Part model, mm, in its own coordinate system. Face numbers are marked on the shaded views. A direction names the side the tool comes from. Give positions to 0.01 mm unless a question says otherwise; leave off trailing zeros. Loops run counter-clockwise (first coordinate to the right, second up) from the corner with the lowest first, then second, coordinate; pieces in that order, holes last. Notation, with made-up numbers: M -38,-16 L 10,-16 A15 ccw 10,1 Z; hole C -17.75,85.25 d3. An arc over 180 degrees is marked long. Answer in a Markdown table with one row per item.
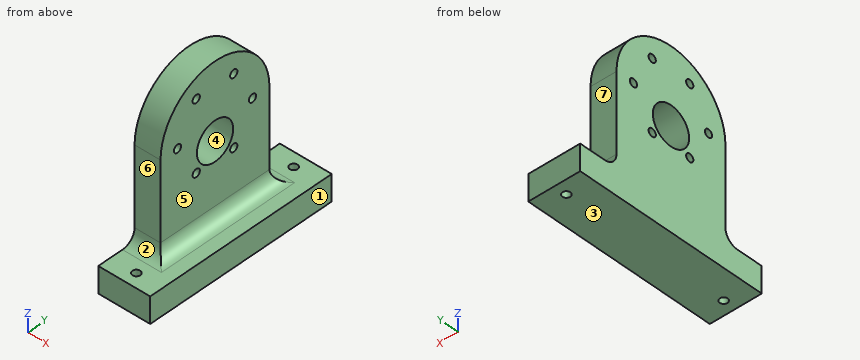
from build123d import *

# Parameters (mm, degrees)
SKETCH1_R           = 7.5
SKETCH1_R_2         = 1.5
BOSS_EXTRUDE1_DEPTH = 10
FILLET1_R           = 5
FILLET2_R           = 5
SKETCH2_W           = 10
SKETCH2_H           = 75
BOSS_EXTRUDE2_DEPTH = 10
FILLET3_R           = 5
SKETCH3_R           = 1.5
CUT_EXTRUDE1_DEPTH  = 10


with BuildPart() as part:
    # Sketch1 → Boss-Extrude1 (new body)
    with BuildSketch(Plane(origin=(0, 0, 0), x_dir=(0, 0, -1), z_dir=(1, 0, 0))):
        with BuildLine():
            Line((0, 0), (35, 0))
            Line((35, 0), (35, -15))
            Line((35, -15), (45, -15))
            Line((45, -15), (45, 60))
            Line((45, 60), (35, 60))
            Line((35, 60), (35, 45))
            Line((35, 45), (0, 45))
            ThreePointArc((0, 45), (-22.5, 22.5), (0, 0))
        make_face()
        with Locations((6.423393759, 22.5)):
            Circle(SKETCH1_R, mode=Mode.SUBTRACT)
        with Locations((13.423393759, 30.25)):
            Circle(SKETCH1_R_2, mode=Mode.SUBTRACT)
        with Locations((0, 38)):
            Circle(SKETCH1_R_2, mode=Mode.SUBTRACT)
        with Locations((-13.423393759, 30.25)):
            Circle(SKETCH1_R_2, mode=Mode.SUBTRACT)
        with Locations((-13.423393759, 14.75)):
            Circle(SKETCH1_R_2, mode=Mode.SUBTRACT)
        with Locations((0, 7)):
            Circle(SKETCH1_R_2, mode=Mode.SUBTRACT)
        with Locations((13.423393759, 14.75)):
            Circle(SKETCH1_R_2, mode=Mode.SUBTRACT)
    extrude(amount=BOSS_EXTRUDE1_DEPTH)

    # Fillet1
    fillet1_edges = [part.edges().sort_by_distance(p)[0] for p in [
        (5, 45, -35),
    ]]
    fillet(fillet1_edges, radius=FILLET1_R)

    # Fillet2
    fillet2_edges = [part.edges().sort_by_distance(p)[0] for p in [
        (5, 0, -35),
    ]]
    fillet(fillet2_edges, radius=FILLET2_R)

    # Sketch2 → Boss-Extrude2 (add)
    with BuildSketch(Plane(origin=(10, 0, 0), x_dir=(0, 0, -1), z_dir=(1, 0, 0))):
        with Locations((40, 22.5)):
            Rectangle(SKETCH2_W, SKETCH2_H)
    extrude(amount=BOSS_EXTRUDE2_DEPTH)

    # Fillet3
    fillet3_edges = [part.edges().sort_by_distance(p)[0] for p in [
        (10, 22.5, -35),
    ]]
    fillet(fillet3_edges, radius=FILLET3_R)

    # Sketch3 → Cut-Extrude1 (cut)
    with BuildSketch(Plane.XY.offset(-35)):
        with Locations((10, -10)):
            Circle(SKETCH3_R)
        with Locations((10, 55)):
            Circle(SKETCH3_R)
    extrude(amount=-CUT_EXTRUDE1_DEPTH, mode=Mode.SUBTRACT)


solid = part.part
(1) Saw through at B-B (x = 6.5). Write the cut outline in (y, z).
Recorded:
| item | result |
|---|---|
| outline | M -15,-45 L 60,-45 L 60,-35 L 50,-35 A5 cw 45,-30 L 45,0 A22.5 ccw 0,0 L 0,-30 A5 cw -5,-35 L -15,-35 Z; hole C 7,0 d3; hole C 14.75,-13.42 d3; hole C 14.75,13.42 d3; hole C 22.5,-6.42 d15; hole C 30.25,-13.42 d3; hole C 30.25,13.42 d3; hole C 38,0 d3 |
(2) Saw through at D-D (z = -27). Write the cut outline in (x, y).
Recorded:
| item | result |
|---|---|
| outline | M 0,0 L 10,0 L 10,45 L 0,45 Z |
(3) Saw through at A-A (y = 22.5). Write the cut outline in (x, z).
Recorded:
| item | result |
|---|---|
| outline | M 0,-45 L 20,-45 L 20,-35 L 15,-35 A5 cw 10,-30 L 10,-13.92 L 0,-13.92 Z; M 0,1.08 L 10,1.08 L 10,22.5 L 0,22.5 Z |
(4) Saw through at C-C (y = -10). Write the cut outline in (x, z), plus the area to 3 significant figures.
Recorded:
| item | result |
|---|---|
| outline | M 0,-45 L 8.5,-45 L 8.5,-35 L 0,-35 Z; M 11.5,-45 L 20,-45 L 20,-35 L 11.5,-35 Z |
| area | 170 mm^2 |
(5) Drill centre lines: line 1 along Y through (x, z) = (10, -43); line 2 along Z through (x, y) = (17.5, 55); line 3 along X through (y, z) = (28, 3). Where is each one in solid material? Low to high.
Recorded:
| item | result |
|---|---|
| line 1 | y = -15 to -11.5, -8.5 to 53.5, 56.5 to 60 |
| line 2 | z = -45 to -35 |
| line 3 | x = 0 to 10 |
(6) Pin check, flat tips, straight feed: pin 1 Ø1.5 at (x, y) = (15, 39.5) entering from +Z; pin 2 Ø5 at (x, y) = (10, 55) entering from -Z; pin 3 Ø3.5 at (y, z) = (38, 0) entering from +X; pin 4 Ø4 at (x, y) = (10, -10) entering from +Z. Stop position of each tip, or through.
Recorded:
| item | result |
|---|---|
| pin 1 | stops at z = -34.94 |
| pin 2 | stops at z = -45 |
| pin 3 | stops at x = 10 |
| pin 4 | stops at z = -35 |
(7) Which spindle directions (+Z, -Z, +X, -X, +Y, -Y) get a long thin tool onto all of the face, cutting with end or side? Do the marked faces 5, 6 and 7. Say none if no direction does.
Recorded:
| item | result |
|---|---|
| face 5 | +Z, +X, +Y, -Y |
| face 6 | +Z, +X, -X, -Y |
| face 7 | +Z, +X, -X, +Y |
(8) Pull direction Z, two halves, no side cores. Call the marked faces 1, 2, 3 and 4: +Z half, -Z half, draft (parallel to the pull), parting line (faces both ways), or undercut.
Recorded:
| item | result |
|---|---|
| face 1 | draft |
| face 2 | +Z half |
| face 3 | -Z half |
| face 4 | undercut |
